Can you work these out from the model? Positions are in its coordinate system, mm. A direction names the side the tool comes from. Coordinates: 2 decimals unless noted, no trailing zeros. Loops run counter-clockwise (first coordinate to the right, second up) from the corner with the lowest first, then second, coordinate; pieces in that order, holes last. Notation, with made-up numbers: M -16.5,-15 L 10.5,-15 A19 ccw 10.5,17 Z; hole C 29,-4 d5. An arc over 180 degrees is marked long. Return JSON: item names as keys, results as strings. Group by question number.
```python
from build123d import *

# Parameters (mm, degrees)
SKETCH2_W           = 350
SKETCH2_H           = 350
BOSS_EXTRUDE1_DEPTH = 20
SKETCH3_R           = 6.35
CUT_EXTRUDE1_DEPTH  = 496.37864306
BOSS_EXTRUDE2_START = 25.4
SKETCH3_3_R         = 9.525
SKETCH3_3_R_2       = 6.35
BOSS_EXTRUDE2_DEPTH = 25.4


with BuildPart() as part:
    # Sketch2 → Boss-Extrude1 (new body)
    with BuildSketch(Plane(origin=(0, 0, 0), x_dir=(1, 0, 0), z_dir=(0, 1, 0))):
        with Locations((175, 175)):
            Rectangle(SKETCH2_W, SKETCH2_H)
    extrude(amount=BOSS_EXTRUDE1_DEPTH)

    # Sketch3 → Cut-Extrude1 (cut, through all)
    with BuildSketch(Plane(origin=(0, 20, 0), x_dir=(1, 0, 0), z_dir=(0, 1, 0))):
        with Locations(Location((175, 175, 0), (0, 0, 270))):
            Circle(SKETCH3_R)
    extrude(amount=-CUT_EXTRUDE1_DEPTH, mode=Mode.SUBTRACT)

    # Sketch3_3 → Boss-Extrude2 (add)
    with BuildSketch(Plane(origin=(0, 20, 0), x_dir=(1, 0, 0), z_dir=(0, 1, 0)).offset(BOSS_EXTRUDE2_START)):
        with Locations(Location((175, 175, 0), (0, 0, 90))):
            Circle(SKETCH3_3_R)
        with Locations(Location((175, 175, 0), (0, 0, 270))):
            Circle(SKETCH3_3_R_2, mode=Mode.SUBTRACT)
    extrude(amount=-BOSS_EXTRUDE2_DEPTH)


solid = part.part
```
1) For faces 1 (the face through (211, 0, -177)), 2 (the face through (168.56, 32.88, -167.98)), which set-ups out of +Z, -Z, +X, -X, +Y, -Y let a thin tool reach every point of the face, with its end or its side?
2) If I drill on line 1 (X direction, y = 15, z = -174); line 2 (X direction, y = 33, z = -175) (3 decimals); line 3 (Y direction, x = 129, z = -325), over which ranges is the centre line in solid material (lowest first)? Write a range as from..to.
3) Suppose I cut it at B-B, the plane z = -175. List the corners of the cut face in (x, y) for me (3 decimals), then the cut area to 3 significant figures.
4) If we mould it in two halves opening along X, with no side actions, what happens to faces 3 (the face through (176.907, 23.018, -168.943)), 4 (the face through (350, 10, -173)), 5 (the face through (0, 10, -173))? For each: +X half, -X half, draft (parallel to the pull), parting line (faces both ways), or undercut.
5) Suppose I cut it at C-C, the plane y = 31. List the corners of the cut face in (x, z) for me (3 decimals).
6) Suppose I cut it at D-D, the plane x = 138. List the corners of the cut face in (y, z) for me, then the cut area to 3 significant figures.
7) Suppose I cut it at A-A, the plane x = 175. List the corners of the cut face in (y, z) for me (3 decimals).
8) For pin 1 (12 mm diameter, centred on x = 300.5, z = -192, fed in from +Y); pin 2 (6 mm diameter, centred on x = 250, z = -241.5, fed in from -Y), each with a flat end and sliding along its axis, tell me the tip position at first contact or that it passes through.
Returned:
{
 "1": {"face 1": "+Z, -Z, +X, -X, -Y", "face 2": "+Y"},
 "2": {"line 1": "x = 0..168.73, 181.27..350", "line 2": "x = 165.475..168.65, 181.35..184.525", "line 3": "y = 0..20"},
 "3": {"outline": "M 0,0 L 168.65,0 L 168.65,45.4 L 165.475,45.4 L 165.475,20 L 0,20 Z; M 181.35,0 L 350,0 L 350,20 L 184.525,20 L 184.525,45.4 L 181.35,45.4 Z", "area": "6,910 mm²"},
 "4": {"face 3": "undercut", "face 4": "+X half", "face 5": "-X half"},
 "5": {"outline": "C 175,-175 d19.05; hole C 175,-175 d12.7"},
 "6": {"outline": "M 0,-350 L 20,-350 L 20,0 L 0,0 Z", "area": "7,000 mm²"},
 "7": {"outline": "M 0,-350 L 20,-350 L 20,-184.525 L 45.4,-184.525 L 45.4,-181.35 L 0,-181.35 Z; M 0,-168.65 L 45.4,-168.65 L 45.4,-165.475 L 20,-165.475 L 20,0 L 0,0 Z"},
 "8": {"pin 1": "stops at y = 20", "pin 2": "stops at y = 0"}
}
